Autodesk Inventor part; units mm, degrees
ref_plane "YZ Plane" through (0, 0, 0) normal (1, 0, 0) x (0, 1, 0)
ref_plane "XZ Plane" through (0, 0, 0) normal (0, 1, 0) x (-1, 0, 0)
ref_plane "XY Plane" through (0, 0, 0) normal (0, 0, 1) x (1, 0, 0)
sketch "Sketch1" plane through (0, 0, 0) normal (0, 1, 0) x (-1, 0, 0)
  line L0 (41.275, 41.275) -> (-41.275, 41.275)
  line L1 (-41.275, 41.275) -> (-41.275, -41.275)
  line L2 (-41.275, -41.275) -> (41.275, -41.275)
  line L3 (41.275, -41.275) -> (41.275, 41.275)
  circle A0 centre (0, 0) radius 44.45 construction
  circle A1 centre (0, 0) radius 39.6875
  line L4 (-41.275, 41.275) -> (41.275, -41.275) construction
  line L5 (41.275, 41.275) -> (-41.275, -41.275) construction
  circle A2 centre (31.4309, 31.4309) radius 2.159
  circle A3 centre (31.4309, -31.4309) radius 2.159
  circle A4 centre (-31.4309, 31.4309) radius 2.159
  circle A5 centre (-31.4309, -31.4309) radius 2.159
  point P0 (0, 0)
  point P1 (0, 0)
  point P2 (0, 0)
  dimension "d0" = 82.55
  dimension "d1" = 82.55
  dimension "d2" = 88.9
  dimension "d3" = 79.375
  dimension "d4" = 4.318
  dimension "d5" = 4.318
  dimension "d6" = 4.318
  dimension "d7" = 4.318
extrude "Extrusion1" add sketch "Sketch1" along normal blind 3.175 contours L3 L2 L1 L0 | A1
sketch "Sketch2" plane through (0, 3.175, 0) normal (0, 1, 0) x (1, 0, 0)
  circle A0 centre (0, 0) radius 39.0525
  circle A1 centre (0, 0) radius 39.6875 construction
  point P0 (0, 0)
  dimension "d10" = 78.105
  dimension "d17" = 79.375
extrude "Extrusion2" add sketch "Sketch2" along normal blind 1.905
fillet "Fillet1" radius 3.175 1 edges at (41.275, 1.5875, 41.275)
fillet "Fillet2" radius 3.175 1 edges at (-41.275, 1.5875, 41.275)
fillet "Fillet3" radius 3.175 1 edges at (41.275, 1.5875, -41.275)
fillet "Fillet4" radius 3.175 1 edges at (-41.275, 1.5875, -41.275)
sketch "Sketch3" plane through (0, 5.08, 0) normal (0, 1, 0) x (1, 0, 0)
  line L0 (0, 24.765) -> (0, -24.765) construction
  line L1 (-23.3045, 0) -> (23.3045, 0) construction
  line L2 (-21.59, -23.0505) -> (21.59, -23.0505) construction
  line L3 (21.59, -23.0505) -> (21.59, 23.0505) construction
  line L4 (21.59, 23.0505) -> (-21.59, 23.0505) construction
  line L5 (-21.59, 23.0505) -> (-21.59, -23.0505) construction
  line L6 (-21.59, -23.0505) -> (21.59, 23.0505) construction
  line L7 (21.59, -23.0505) -> (-21.59, 23.0505) construction
  line L8 (-27.7495, -27.7495) -> (27.7495, 27.7495) construction
  line L9 (27.7495, -27.7495) -> (-27.7495, 27.7495) construction
  line L10 (-14.8242, 24.765) -> (14.1532, 24.765)
  line L11 (-14.8242, 24.765) -> (-23.3045, 15.7122)
  line L12 (23.3045, 16.1923) -> (23.3045, -15.7122)
  line L13 (23.3045, 16.1923) -> (14.1532, 24.765)
  line L14 (14.8242, -24.765) -> (-14.1532, -24.765)
  line L15 (14.8242, -24.765) -> (23.3045, -15.7122)
  line L16 (-23.3045, -16.1923) -> (-23.3045, 15.7122)
  line L17 (-23.3045, -16.1923) -> (-14.1532, -24.765)
  point P0 (0, 0)
  point P1 (0, 0)
  dimension "d20" = 43.18
  dimension "d21" = 46.101
extrude "Extrusion3" cut sketch "Sketch3" against normal through all
hole "Hole1" at (-21.59, 5.08, -23.0505) at (21.59, 5.08, 23.0505) at (21.59, 5.08, -23.0505) at (-21.59, 5.08, 23.0505) direction (0, -1, 0) diameter 3.175 end through all
properties part number "ka51a-instrument-mount"
Build history of the part. All positions in model axes, mm. A direction names the side the tool comes from. Coordinates: 2 decimals unless noted, no trailing zeros. Write each loop counter-clockwise with the first axis right and the second up, starting at its lowest first coordinate (ties: lowest second). Pieces come first, ordered by that corner, then holes.
1. Drop flat-ended pins along their axis: pin 1 (3 mm diameter, centred on x = -21.59, z = 23.05, fed in from +Y); pin 2 (3.5 mm diameter, centred on x = 21.59, z = -23.05, fed in from -Y); pin 3 (5.5 mm diameter, centred on x = 31.43, z = -31.43, fed in from +Y) (3 decimals). Give the stop position or say it passes through.
Answer block:
pin 1: passes through
pin 2: stops at y = 0
pin 3: stops at y = 3.175
2. Band-saw the part on B-B, the plane x = 0. Give the cut face in (y, z) (1 decimal).
Answer block:
outline: (0, -41.3) - (3.2, -41.3) - (3.2, -39.1) - (5.1, -39.1) - (5.1, -24.8) - (0, -24.8) - close; (0, 24.8) - (5.1, 24.8) - (5.1, 39.1) - (3.2, 39.1) - (3.2, 41.3) - (0, 41.3) - close
3. Band-saw the part on A-A, the plane z = 0. Give the cut face in (x, y) (1 decimal), and give its area (3 significant figures).
Answer block:
outline: (-41.3, 0) - (-23.3, 0) - (-23.3, 5.1) - (-39.1, 5.1) - (-39.1, 3.2) - (-41.3, 3.2) - close; (23.3, 0) - (41.3, 0) - (41.3, 3.2) - (39.1, 3.2) - (39.1, 5.1) - (23.3, 5.1) - close
area: 174 mm2
4. Band-saw the part on D-D, the plane x = -21.59. Give the cut face in (y, z) (3 decimals).
Answer block:
outline: (0, -41.275) - (3.175, -41.275) - (3.175, -32.542) - (5.08, -32.542) - (5.08, -24.638) - (0, -24.638) - close; (0, -21.463) - (5.08, -21.463) - (5.08, -17.542) - (0, -17.542) - close; (0, 17.798) - (5.08, 17.798) - (5.08, 21.463) - (0, 21.463) - close; (0, 24.638) - (5.08, 24.638) - (5.08, 32.542) - (3.175, 32.542) - (3.175, 41.275) - (0, 41.275) - close
5. Pull direction X, two halves, no side cores. Call faces 3 (the cylindrical face through (40.32, 1.61, 40.37)), 4 (the cylindrical face through (-20.624, 2.504, -24.31)), 5 (the flat face through (15, 3.175, 37)), 6 (the cylindrical face through (29.37, 1.57, -32.08)): released by +X, released by -X, zero draft, split by the parting line, or undercut.
Answer block:
face 3: released by +X
face 4: undercut
face 5: zero draft
face 6: undercut
6. Band-saw the part on C-C, the plane y = 1.2. Give the number of separate pieces and of enclosed holes in the cut face, and give its area (3 significant figures).
Answer block:
separate pieces: 1
enclosed holes: 9
area: 4,560 mm2
7. Drill centre lines: probe 1 along X at (y, z) = (0.85, -12) (1 decimal); probe 2 along X at (y, z) = (4.2, -8.5); probe 3 along Z at (x, y) = (12, 0.6) (3 decimals). Where is each one in solid material? Low to high.
Answer block:
probe 1: x = -41.3 to -23.3, 23.3 to 41.3
probe 2: x = -38.12 to -23.3, 23.3 to 38.12
probe 3: z = -41.275 to -24.765, 24.765 to 41.275
8. 3-axis set-ups, long thin cutter, end or side, ignore diameter. For faces 1 (the flat face through (-1, 5.08, 25)), 2 (the flat face through (-23.304, 3, 0)): which of +Z, -Z, +X, -X, +Y, -Y reach the whole face in a straight line?
Answer block:
face 1: +Z, -Z, +X, -X, +Y
face 2: +Y, -Y
